Autodesk Inventor part; units mm, degrees
ref_plane "YZ Plane" through (0, 0, 0) normal (1, 0, 0) x (0, 1, 0)
ref_plane "XZ Plane" through (0, 0, 0) normal (0, 1, 0) x (-1, 0, 0)
ref_plane "XY Plane" through (0, 0, 0) normal (0, 0, 1) x (1, 0, 0)
sketch "Sketch1" plane through (0, 0, 0) normal (0, 1, 0) x (-1, 0, 0)
  line L0 (17.7305, 21.844) -> (-22.2695, 21.844)
  line L1 (-22.2695, 21.844) -> (-22.2695, -18.156)
  line L2 (-22.2695, -18.156) -> (17.7305, -18.156)
  line L3 (17.7305, -18.156) -> (17.7305, 21.844)
  line L4 (22.8105, 26.924) -> (-27.3495, 26.924)
  line L5 (-27.3495, 26.924) -> (-27.3495, -23.236)
  line L6 (-27.3495, -23.236) -> (22.8105, -23.236)
  line L7 (22.8105, -23.236) -> (22.8105, 26.924)
  point P0 (0, 0)
  dimension "d0" = 40
  dimension "d1" = 40
  dimension "d2" = 5.08
  dimension "d3" = 5.08
  dimension "d4" = 5.08
  dimension "d5" = 5.08
extrude "Extrusion1" add sketch "Sketch1" along normal blind 7.62
sketch "Sketch2" plane through (0, 0, 0) normal (0, -1, 0) x (1, 0, 0)
  line L0 (37.5095, 37.084) -> (-32.9705, 37.084)
  line L1 (-32.9705, 37.084) -> (-32.9705, -33.396)
  line L2 (-32.9705, -33.396) -> (37.5095, -33.396)
  line L3 (37.5095, -33.396) -> (37.5095, 37.084)
  line L4 (-22.8105, 26.924) -> (27.3495, 26.924)
  line L5 (27.3495, 26.924) -> (27.3495, -23.236)
  line L6 (-22.8105, -23.236) -> (-22.8105, 26.924)
  line L7 (27.3495, -23.236) -> (-22.8105, -23.236)
  point P0 (0, 0)
  dimension "d8" = 10.16
  dimension "d9" = 10.16
  dimension "d10" = 10.16
  dimension "d11" = 10.16
extrude "Extrusion2" add sketch "Sketch2" along normal blind 5.08 contours L3 L2 L1 L0 | L4 L5 L7 L6
sketch "Sketch3" plane through (0, 0, 0) normal (0, 1, 0) x (1, 0, 0)
  line L0 (-32.9705, 33.396) -> (37.5095, 33.396)
  line L1 (-32.9705, -37.084) -> (-32.9705, 33.396)
  line L2 (37.5095, 33.396) -> (37.5095, -37.084)
  line L3 (37.5095, -37.084) -> (-32.9705, -37.084)
  point P0 (0, 0)
  point P1 (-27.8905, 28.316)
  point P2 (32.4295, 28.3337)
  point P3 (31.8578, -32.004)
  point P4 (-27.206, -31.7168)
  dimension "d14" = 5.08
  dimension "d15" = 5.08
  dimension "d16" = 5.08
  dimension "d17" = 5.08
hole "Hole1" at (-27.8905, 0, -28.316) at (32.4295, 0, -28.3337) at (31.8578, 0, 32.004) at (-27.206, 0, 31.7168) direction (0, -1, 0) diameter 5.08 depth 25.4 tip angle 118 countersink diameter 9.525 countersink angle 82
sketch "Sketch4" plane through (0, 0, 0) normal (0, 1, 0) x (1, 0, 0)
  line L0 (-17.7305, 18.156) -> (22.2695, 18.156)
  line L1 (22.2695, -21.844) -> (-17.7305, -21.844)
  line L2 (22.2695, -21.844) -> (22.2695, 18.156)
  line L3 (-17.7305, 18.156) -> (-17.7305, -21.844)
  point P0 (0, 0)
  point P1 (-12.2305, 12.656)
  point P2 (16.7695, 12.656)
  point P3 (16.7695, -16.344)
  point P4 (-12.7285, -16.7964)
  dimension "d25" = 29
  dimension "d26" = 29
  dimension "d27" = 5.5
  dimension "d28" = 5.5
  dimension "d29" = 5.5
  dimension "d30" = 5.5
hole "Hole2" at (-12.2305, 0, -12.656) at (16.7695, 0, -12.656) at (16.7695, 0, 16.344) at (-12.7285, 0, 16.7964) direction (0, -1, 0) diameter 3.5 depth 25.4 tip angle 118
sketch "Sketch5" plane through (0, 7.62, 0) normal (0, 1, 0) x (1, 0, 0)
  line L0 (-7.5705, -40.5496) -> (12.1095, -40.5496)
  line L1 (12.1095, -40.5496) -> (12.1095, -14.6017)
  line L2 (12.1095, -14.6017) -> (-7.5705, -14.6017)
  line L3 (-7.5705, -14.6017) -> (-7.5705, -40.5496)
  line L4 (-22.8105, 23.236) -> (-22.8105, -26.924)
  line L5 (27.3495, -26.924) -> (27.3495, 23.236)
  point P0 (0, 0)
  dimension "d38" = 15.24
  dimension "d39" = 15.24
extrude "Extrusion3" cut sketch "Sketch5" against normal blind 6.35
properties part number "PigeonIMUMount"
Check sheet for the modelled part. Datum: model origin and axes. Units: mm. A direction names the side the tool comes from. Give positions to 0.01 mm unless a question says otherwise; leave off trailing zeros. Loops run counter-clockwise (first coordinate to the right, second up) from the corner with the lowest first, then second, coordinate; pieces in that order, holes last. Notation, with made-up numbers: M -25,-38.75 L 29,-38.75 A24 cw 29,-4.75 Z; hole C 34,30 d8. An arc over 180 degrees is marked long. Return JSON: item names as keys, results as strings. Group by question number.
1. Cross-section at C-C on x = 14. Record the boundary of the cut face in (y, z), plus the area to 3 significant figures.
2. Go/stop test with flat-tipped pins: pin 1 (2 mm diameter, centred on x = 11, y = 2.5, fed in from -Z); pin 2 (6 mm diameter, centred on y = 4, z = 10.5, fed in from -X); pin 3 (1 mm diameter, centred on y = 2, z = -11, fed in from +X). Record where each tip stops, or that it passes through.
3. Tool access check on faces 1 (the flat face through (27.35, 4, 2)), 2 (the flat face through (2, 0, 2)), 3 (the flat face through (2, -5.08, 2)). Record the directions out of +Z, -Z, +X, -X, +Y, -Y that give a thin tool (end or side, any length) a straight path to the whole face; none if there is none.
4. Mould release check, pull along X, two halves, no side actions. Record for faces 4 (the flat face through (2.4, 7.62, -18.5)), 5 (the flat face through (-7.57, 4, 24)), 6 (the flat face through (-32.97, -3, 2)), 7 (the cylindrical face through (-11.66, -2.58, 15.41)): released by +X, released by -X, zero draft, split by the parting line, or undercut.
5. Thickness scan on L1, parallel to X at y = 4.5, z = 10; L2, parallel to Z at x = 15.5, y = 6.5; L3, parallel to X at y = -0.5, z = -25.5. Record the ranges inside material, lowest first.
6. Cross-section at B-B on y = -4. State how many separate pieces and enclosed holes the cut face has, plus the area to 3 significant figures.
7. Cross-section at D-D on z = 17. Record the boundary of the cut face in (x, y), plus the area to 3 significant figures.
8. Cross-section at A-A on z = 25. Record the boundary of the cut face in (x, y).
Return value:
{
 "1": {"outline": "M -5.08,-33.4 L 0,-33.4 L 0,-23.24 L 7.62,-23.24 L 7.62,-18.16 L 0,-18.16 L 0,21.84 L 7.62,21.84 L 7.62,26.92 L 0,26.92 L 0,37.08 L -5.08,37.08 Z", "area": "435 mm^2"},
 "2": {"pin 1": "z = -23.24", "pin 2": "x = -22.81", "pin 3": "x = 27.35"},
 "3": {"face 1": "+Z, -Z, +X, +Y", "face 2": "+Y", "face 3": "+Z, -Z, +X, -X, -Y"},
 "4": {"face 4": "zero draft", "face 5": "undercut", "face 6": "released by -X", "face 7": "undercut"},
 "5": {"L1": "-22.81 to -17.73, 22.27 to 27.35", "L2": "-23.24 to -18.16, 21.84 to 26.92", "L3": "-32.97 to -31.18, -24.6 to 29.16, 35.7 to 37.51"},
 "6": {"separate pieces": "1", "enclosed holes": "8", "area": "4,850 mm^2"},
 "7": {"outline": "M -32.97,-5.08 L -14.47,-5.08 L -14.47,0 L -17.73,0 L -17.73,7.62 L -22.81,7.62 L -22.81,0 L -32.97,0 Z; M -10.99,-5.08 L 15.15,-5.08 L 15.15,0 L -10.99,0 Z; M 18.39,-5.08 L 37.51,-5.08 L 37.51,0 L 27.35,0 L 27.35,7.62 L 22.27,7.62 L 22.27,0 L 18.39,0 Z", "area": "401 mm^2"},
 "8": {"outline": "M -32.97,-5.08 L 37.51,-5.08 L 37.51,0 L 27.35,0 L 27.35,7.62 L 12.11,7.62 L 12.11,1.27 L -7.57,1.27 L -7.57,7.62 L -22.81,7.62 L -22.81,0 L -32.97,0 Z"}
}
